from build123d import *

# Parameters (mm, degrees)
SKETCH1_R           = 31.496
SKETCH1_R_2         = 12.7
BOSS_EXTRUDE1_DEPTH = 12.7
BOSS_EXTRUDE2_START = -5.08
SKETCH3_R           = 1.397
BOSS_EXTRUDE2_DEPTH = 6.35


with BuildPart() as part:
    # Sketch1 → Boss-Extrude1 (new body)
    with BuildSketch(Plane(origin=(0, 0, 0), x_dir=(1, 0, 0), z_dir=(0, 1, 0))):
        with Locations(Location((0, 0, 0), (0, 0, 270))):
            Circle(SKETCH1_R)
        with Locations(Location((0, 0, 0), (0, 0, 270))):
            Circle(SKETCH1_R_2, mode=Mode.SUBTRACT)
    extrude(amount=BOSS_EXTRUDE1_DEPTH)

    # Sketch3 → Boss-Extrude2 (add)
    with BuildSketch(Plane.XY.offset(-12.7).offset(BOSS_EXTRUDE2_START)):
        with Locations((0, 6.35)):
            Circle(SKETCH3_R)
    boss_extrude2 = extrude(amount=BOSS_EXTRUDE2_DEPTH)

    # Mirror1: Boss-Extrude2 across plane
    add(boss_extrude2.mirror(Plane.XY))


solid = part.part
Could you check a few things on this model? Use its own coordinates, in mm. A direction names the side the tool comes from. Give positions to 0.01 mm unless a question says otherwise; leave off trailing zeros. Order: outer loops, then holes, each group sorted by start corner. A loop starts at its lowest first (then second) coordinate and runs counter-clockwise, first axis right, second up.
1. Suppose I cut it at B-B (z = -10.5). Write out the boundary of the cut face in (x, y), plus the area to 3 significant figures.
Answers below:
outline: (-29.69, 0) - (-7.14, 0) - (-7.14, 12.7) - (-29.69, 12.7) - close; (7.14, 0) - (29.69, 0) - (29.69, 12.7) - (7.14, 12.7) - close
area: 573 mm2
2. Suppose I cut it at A-A (x = 0). Write out the boundary of the cut face in (y, z), plus the area to 3 significant figures.
Answers below:
outline: (0, -31.5) - (12.7, -31.5) - (12.7, -12.7) - (7.75, -12.7) - (7.75, -11.43) - (4.95, -11.43) - (4.95, -12.7) - (0, -12.7) - close; (0, 12.7) - (4.95, 12.7) - (4.95, 11.43) - (7.75, 11.43) - (7.75, 12.7) - (12.7, 12.7) - (12.7, 31.5) - (0, 31.5) - close
area: 485 mm2
3. Which directions (+Z, -Z, +X, -X, +Y, -Y) give clear straight access to the entire face, cutting with the end or side of a thin tool? Please do faces 4 (the flat face through (0, 12.7, 14)), 5 (the flat face through (0, 6, -11.43)), 6 (the cylindrical face through (-1.396, 6.411, 12.074)).
Answers below:
face 4: +Z, -Z, +X, -X, +Y
face 5: +Y, -Y
face 6: none
4. I need wall thicknesses on L1, parallel to X at y = 6, z = 0; L2, parallel to X at y = 10.25, z = 3.5; L3, parallel to Z at x = -16.5, y = 10.5. Which ranges of each line are inside material? Lowest first, please.
Answers below:
L1: x = -31.5 to -12.7, 12.7 to 31.5
L2: x = -31.3 to -12.21, 12.21 to 31.3
L3: z = -26.83 to 26.83
5. Suppose I cut it at C-C (y = 6.35). Write out the boundary of the cut face in (x, z), plus the area to 3 significant figures.
Answers below:
outline: circle Ø62.99 at (0, 0); hole (-1.4, -12.62) - (-1.4, -11.43) - (1.4, -11.43) - (1.4, -12.62) arc R12.7 ccw to (1.4, 12.62) - (1.4, 11.43) - (-1.4, 11.43) - (-1.4, 12.62) arc R12.7 ccw to start
area: 2,620 mm2
6. Thinking about a two-plate mould opening in Z: for faces 1 (the cylindrical face through (-30.747, 6.261, -6.828)), 2 (the cylindrical face through (-1.396, 6.411, -12.075)), 3 (the flat face through (0, 0, 14)), which applies, +Z half, -Z half, draft (parallel to the pull), parting line (faces both ways), or undercut?
Answers below:
face 1: parting line
face 2: undercut
face 3: draft
7. Suppose I cut it at D-D (x = -7). Write out the boundary of the cut face in (y, z), plus the area to 3 significant figures.
Answers below:
outline: (0, -30.71) - (12.7, -30.71) - (12.7, -10.6) - (0, -10.6) - close; (0, 10.6) - (12.7, 10.6) - (12.7, 30.71) - (0, 30.71) - close
area: 511 mm2
8. For pin 1 (1.5 mm diameter, centred on y = 4.5, z = -4.5, fed in from -X); pin 2 (1 mm diameter, centred on y = 5.5, z = -14.5, fed in from +X), each with a flat end and sliding along its axis, tell me the tip position at first contact or that it passes through.
Answers below:
pin 1: stops at x = -31.27
pin 2: stops at x = 28.21
